```python
from build123d import *
from OCP.BRepFilletAPI import BRepFilletAPI_MakeChamfer

# Parameters (mm, degrees)
BOSS_EXTRUDE1_DEPTH      = 88.9
CUT_EXTRUDE2_DEPTH       = 130.67066939
CUT_EXTRUDE2_DEPTH_BACK  = 130.67066939
SKETCH12_W               = 127
SKETCH12_H               = 127
CUT_EXTRUDE3_START       = -3.175
SKETCH11_W               = 165.1
SKETCH11_H               = 165.1
CUT_EXTRUDE3_DEPTH       = 127.49566939
CUT_EXTRUDE4_START       = 3.175
SKETCH11_2_W             = 165.1
SKETCH11_2_H             = 165.1
CUT_EXTRUDE4_DEPTH       = 127.49566939
FILLET3_R                = 12.7
F_9_16_12_TAPPED_HOLE1_D = 12.30376
CHAMFER2_SIZE            = 1.27
CHAMFER2_SIZE2           = 1.132534886
CHAMFER2_SIZE2_2         = 1.47384677


with BuildPart() as part:
    # Sketch1 → Boss-Extrude1 (new, symmetric)
    with BuildSketch(Plane(origin=(0, 0, 0), x_dir=(-1, 0, 0), z_dir=(0, 1, 0))):
        Polygon((31.75, -88.9), (-31.75, -88.9), (-8.466666667, 88.9), (8.466666667, 88.9), align=None)
    extrude(amount=BOSS_EXTRUDE1_DEPTH, both=True)

    # Sketch12 → Cut-Extrude2 (cut, two sides: drawn at the far end of the back side and taken through both)
    with BuildSketch(Plane.YZ.offset(-CUT_EXTRUDE2_DEPTH_BACK)):
        Rectangle(SKETCH12_W, SKETCH12_H)
    extrude(amount=CUT_EXTRUDE2_DEPTH + CUT_EXTRUDE2_DEPTH_BACK, mode=Mode.SUBTRACT)

    # Sketch11 → Cut-Extrude3 (cut, through all)
    with BuildSketch(Plane.YZ.offset(CUT_EXTRUDE3_START)):
        Rectangle(SKETCH11_W, SKETCH11_H)
    extrude(amount=-CUT_EXTRUDE3_DEPTH, mode=Mode.SUBTRACT)

    # Sketch11<2> → Cut-Extrude4 (cut, through all)
    with BuildSketch(Plane.YZ.offset(CUT_EXTRUDE4_START)):
        Rectangle(SKETCH11_2_W, SKETCH11_2_H)
    extrude(amount=CUT_EXTRUDE4_DEPTH, mode=Mode.SUBTRACT)

    # Fillet3
    fillet3_edges = [part.edges().sort_by_distance(p)[0] for p in [
        (0, -63.5, 63.5),
        (0, 63.5, 63.5),
        (0, -63.5, -63.5),
        (0, 63.5, -63.5),
    ]]
    fillet(fillet3_edges, radius=FILLET3_R)

    # 9/16-12 Tapped Hole1 (through all)
    with Locations(Plane(origin=(0, 0, -88.9), x_dir=(1, 0, 0), z_dir=(0, 0, -1))):
        with Locations((-17.4625, 60.325), (17.4625, 60.325), (17.4625, -60.325), (-17.4625, -60.325)):
            Hole(F_9_16_12_TAPPED_HOLE1_D / 2)

    # Chamfer2: one chamfer whose edges measure the first distance from different faces: ONE call of the kernel's chamfer builder (chamfer() names one face for all edges)
    chamfer2_edges_1 = [part.edges().sort_by_distance(p)[0] for p in [
        (-3.175, -63.5, 0),
        (3.175, 0, -63.5),
        (-3.175, 0, -63.5),
        (3.175, 59.780256121, 59.780256121),
        (-3.175, 59.780256121, 59.780256121),
        (3.175, -59.780256121, 59.780256121),
        (-3.175, -59.780256121, 59.780256121),
        (3.175, -59.780256121, -59.780256121),
        (-3.175, -59.780256121, -59.780256121),
        (3.175, 59.780256121, -59.780256121),
        (-3.175, 59.780256121, -59.780256121),
        (0, 88.9, -88.9),
        (20.108333333, 88.9, 0),
        (-20.108333333, -82.55, 0),
        (-20.108333333, 82.55, 0),
        (0, 88.9, 88.9),
        (20.108333333, -88.9, 0),
        (0, -88.9, -88.9),
        (-20.108333333, -88.9, 0),
        (0, -88.9, 88.9),
        (20.108333333, -82.55, 0),
        (20.108333333, 82.55, 0),
        (-20.108333333, 88.9, 0),
        (3.175, 0, 63.5),
        (-3.175, 0, 63.5),
        (3.175, 63.5, 0),
        (-3.175, 63.5, 0),
        (3.175, -63.5, 0),
    ]]
    chamfer2_edges_2 = [part.edges().sort_by_distance(p)[0] for p in [
        (-9.298214286, 0, 82.55),
    ]]
    chamfer2_side_2 = [part.faces().sort_by_distance(p)[0] for p in [
        (-8.794551937, 0, 86.396148844),
    ]]
    chamfer2_edges_3 = [part.edges().sort_by_distance(p)[0] for p in [
        (-30.918452381, 0, -82.55),
        (-8.466666667, 0, 88.9),
    ]]
    chamfer2_side_3 = [part.faces().sort_by_distance(p)[0] for p in [
        (-8.794551937, 0, 86.396148844),
    ]]
    chamfer2_edges_4 = [part.edges().sort_by_distance(p)[0] for p in [
        (30.918452381, 0, -82.55),
    ]]
    chamfer2_side_4 = [part.faces().sort_by_distance(p)[0] for p in [
        (20.108333333, -86.374771424, 0),
    ]]
    chamfer2_edges_5 = [part.edges().sort_by_distance(p)[0] for p in [
        (9.298214286, 0, 82.55),
        (31.75, 0, -88.9),
    ]]
    chamfer2_side_5 = [part.faces().sort_by_distance(p)[0] for p in [
        (20.108333333, -86.374771424, 0),
    ]]
    chamfer2_edges_6 = [part.edges().sort_by_distance(p)[0] for p in [
        (8.466666667, 0, 88.9),
    ]]
    chamfer2_side_6 = [part.faces().sort_by_distance(p)[0] for p in [
        (0, 0, 88.9),
    ]]
    chamfer2_edges_7 = [part.edges().sort_by_distance(p)[0] for p in [
        (-31.75, 0, -88.9),
    ]]
    chamfer2_side_7 = [part.faces().sort_by_distance(p)[0] for p in [
        (0, 0, -88.9),
    ]]
    chamfer2 = BRepFilletAPI_MakeChamfer(part.part.solid().wrapped)
    for e in chamfer2_edges_1:
        chamfer2.Add(CHAMFER2_SIZE, e.wrapped)
    for e in chamfer2_edges_2:
        chamfer2.Add(CHAMFER2_SIZE, CHAMFER2_SIZE2, e.wrapped, chamfer2_side_2[0].wrapped)  # the first distance lies on this face
    for e in chamfer2_edges_3:
        chamfer2.Add(CHAMFER2_SIZE, CHAMFER2_SIZE2_2, e.wrapped, chamfer2_side_3[0].wrapped)  # the first distance lies on this face
    for e in chamfer2_edges_4:
        chamfer2.Add(CHAMFER2_SIZE, CHAMFER2_SIZE2_2, e.wrapped, chamfer2_side_4[0].wrapped)  # the first distance lies on this face
    for e in chamfer2_edges_5:
        chamfer2.Add(CHAMFER2_SIZE, CHAMFER2_SIZE2, e.wrapped, chamfer2_side_5[0].wrapped)  # the first distance lies on this face
    for e in chamfer2_edges_6:
        chamfer2.Add(CHAMFER2_SIZE, CHAMFER2_SIZE2_2, e.wrapped, chamfer2_side_6[0].wrapped)  # the first distance lies on this face
    for e in chamfer2_edges_7:
        chamfer2.Add(CHAMFER2_SIZE, CHAMFER2_SIZE2, e.wrapped, chamfer2_side_7[0].wrapped)  # the first distance lies on this face
    add(Compound.cast(chamfer2.Shape()), mode=Mode.REPLACE)


solid = part.part
```
Geometry check sheet. Reference: the model listing, model coordinates, mm. A direction names the side the tool comes from. Give positions to 0.01 mm unless a question says otherwise; leave off trailing zeros. Loops run counter-clockwise (first coordinate to the right, second up) from the corner with the lowest first, then second, coordinate; pieces in that order, holes last. Notation, with made-up numbers: M 30,44.25 L 75,44.25 A19 cw 75,77.25 Z; hole C -7,58.5 d8. An arc over 180 degrees is marked long. Write item = value, one per line. Start each with the question number.
1. Thickness scan on probe 1 along Y at (x, z) = (6.5, 42). Record the ranges inside material, lowest first.
2. Section check C-C, the plane y = 70.5. Enter the section's corners in (x, z) (3 decimals), plus the area to 3 significant figures.
3. Section check B-B, the plane z = -20. Enter the section's corners in (x, y) (3 decimals), plus the area to 3 significant figures.
4. Draft check along Z on faces 1 (the face through (2.13, 59.84, -60.04)), 2 (the face through (-19.213, -83.976, 6.838)), 3 (the face through (0, 88.9, -18)). Enter one of: +Z half, -Z half, draft (parallel to the pull), parting line (faces both ways), or undercut.
5. Tool access check on faces 4 (the face through (0.03, -59.68, 59.88)), 5 (the face through (-13, 82.55, -20)), 6 (the face through (0, 1, -88.9)), 7 (the face through (13, -82.55, -20)). Record the directions out of +Z, -Z, +X, -X, +Y, -Y that give a thin tool (end or side, any length) a straight path to the whole face; none if there is none.
6. Go/stop test with flat-tipped pins: P1, Ø10, axis at x = 17.46, y = -60.32, coming from the -Z side; P2, Ø21, axis at x = -21.5, z = -5, coming from the -Y side; P3, Ø1, axis at x = 10.5, y = -51.5, coming from the +Z side. Record where each tip stops, or that it passes through.
7. Section check D-D, the plane x = 19. Enter the section's corners in (y, z), plus the area to 3 significant figures.
8. Section check A-A, the plane y = -34. Enter the section's corners in (x, z) (3 decimals).
Values follow:
q1.probe_1 = -88.9 to -82.55, 82.55 to 88.9
q2.outline = M -31.603,-87.777 L -30.48,-88.9 L 30.617,-88.9 L 31.585,-87.641 L 31.083,-83.809 L 29.445,-82.55 L 3.175,-82.55 L 3.175,82.55 L 8.166,82.55 L 9.133,83.809 L 8.658,87.439 L 7.197,88.9 L -6.993,88.9 L -8.632,87.641 L -9.133,83.809 L -8.166,82.55 L -3.175,82.55 L -3.175,-82.55 L -29.445,-82.55 L -31.083,-83.809 Z
q2.area = 1,550 mm^2
q3.outline = M -22.727,-87.63 L -21.447,-88.9 L 21.447,-88.9 L 22.727,-87.63 L 22.727,-83.82 L 21.447,-82.55 L 3.175,-82.55 L 3.175,-64.77 L 1.905,-63.5 L -1.905,-63.5 L -3.175,-64.77 L -3.175,-82.55 L -21.447,-82.55 L -22.727,-83.82 Z; M -22.727,83.82 L -21.447,82.55 L -3.175,82.55 L -3.175,64.77 L -1.905,63.5 L 1.905,63.5 L 3.175,64.77 L 3.175,82.55 L 21.447,82.55 L 22.727,83.82 L 22.727,87.63 L 21.447,88.9 L -21.447,88.9 L -22.727,87.63 Z
q3.area = 809 mm^2
q4.face_1 = undercut
q4.face_2 = +Z half
q4.face_3 = draft
q5.face_4 = +X, -X
q5.face_5 = -X
q5.face_6 = -Z, +X, -X, +Y, -Y
q5.face_7 = +X
q6.P1 = through
q6.P2 = -88.9
q6.P3 = -82.55
q7.outline = M -88.9,-87.63 L -87.63,-88.9 L -66.28,-88.9 L -66.28,-82.55 L -82.55,-82.55 L -82.55,-1.32 L -83.82,8.46 L -87.63,8.46 L -88.9,-1.32 Z; M -54.37,-88.9 L 54.37,-88.9 L 54.37,-82.55 L -54.37,-82.55 Z; M 66.28,-88.9 L 87.63,-88.9 L 88.9,-87.63 L 88.9,-1.32 L 87.63,8.46 L 83.82,8.46 L 82.55,-1.32 L 82.55,-82.55 L 66.28,-82.55 Z
q7.area = 2,110 mm^2
q8.outline = M -31.603,-87.777 L -30.48,-88.9 L 30.617,-88.9 L 31.585,-87.641 L 31.083,-83.809 L 29.445,-82.55 L 3.175,-82.55 L 3.175,-64.77 L 1.905,-63.5 L -1.905,-63.5 L -3.175,-64.77 L -3.175,-82.55 L -29.445,-82.55 L -31.083,-83.809 Z; M -9.133,83.809 L -8.166,82.55 L -3.175,82.55 L -3.175,64.77 L -1.905,63.5 L 1.905,63.5 L 3.175,64.77 L 3.175,82.55 L 8.166,82.55 L 9.133,83.809 L 8.658,87.439 L 7.197,88.9 L -6.993,88.9 L -8.632,87.641 Z
